Input: part model. Units: mm. Frame: model coordinates. Give positions to 0.01 mm unless a question says otherwise; leave off trailing zeros. Loops run counter-clockwise (first coordinate to the right, second up) from the corner with the lowest first, then second, coordinate; pieces in that order, holes last. Notation, with made-up numbers: M -30.75,-31 L 21.25,-31 A22 cw 21.25,-7 Z; hole C -0.5,11 d5. An arc over 180 degrees is marked long. Use CSV: the item, a comma, the result in double quotes. Start each with the question number.
Q1. Pin query (flat end, axial travel): pin 1 (1.1 mm diameter, centred on x = 0, z = 86.5, fed in from +Y); pin 2 (1.1 mm diameter, centred on y = -0.5, z = 83.5, fed in from +X); pin 3 (1.8 mm diameter, centred on x = 0, z = 88.5, fed in from -Y). Return the tip coordinate at first contact, or that it passes through.
Q2. Section A-A, the plane x = 0. Output: boundary loops of the cut face in (y, z).
Q3. Material intervals for line 1 along Y through (x, z) = (0, 107.5); line 2 along Y through (x, z) = (5.5, 63.5); line 3 along X through (y, z) = (3.25, 27), sorted ascending.
Autodesk Inventor part; units mm, degrees
ref_plane "Start Plane" through (0, 0, 10.031) normal (0, 0, 1) x (1, 0, 0)
ref_plane "End Plane" through (0, 0, 139.969) normal (0, 0, 1) x (1, 0, 0)
ref_plane "Work Plane6" through (-500, 9, 10.031) normal (0, 0, -1) x (-1, 0, 0)
ref_plane "Start Plane" through (0, 0, 10.031) normal (0, 0, 1) x (1, 0, 0)
ref_plane "End Plane" through (0, 0, 139.969) normal (0, 0, 1) x (1, 0, 0)
sketch "Sketch" plane through (0, 0, 0) normal (0, 0, 1) x (1, 0, 0)
  line L0 (0, 0) -> (2.5, 0) construction
  line L1 (0, 0) -> (0, 2.5) construction
  line L2 (0, 4) -> (0, -4) construction
  line L3 (0, 4) -> (1.7574, 4)
  arc A0 (1.7574, 4) -> (3.1716, 4.5858) centre (1.7574, 6) ccw
  line L4 (3.1716, 4.5858) -> (5.7322, 7.1464)
  line L5 (-4, 0) -> (4, 0) construction
  line L6 (4, 0) -> (4, 1.7574)
  arc A1 (4.5858, 3.1716) -> (4, 1.7574) centre (6, 1.7574) ccw
  line L7 (4.5858, 3.1716) -> (7.1464, 5.7322)
  line L8 (0, 0) -> (10, 10) construction
  line L9 (0, 0) -> (19.6827, 0) construction
  arc A2 (8, 5.3787) -> (7.1464, 5.7322) centre (7.5, 5.3787) ccw
  line L10 (8, 5.3787) -> (8, 3.5)
  arc A3 (8, 3.5) -> (8.5, 3) centre (8.5, 3.5) ccw
  line L11 (8.5, 3) -> (9.5, 3)
  arc A4 (9.5, 3) -> (10, 3.5) centre (9.5, 3.5) ccw
  line L12 (10, 3.5) -> (10, 9)
  line L13 (10, 9) -> (10, 10) construction
  arc A5 (5.7322, 7.1464) -> (5.3787, 8) centre (5.3787, 7.5) ccw
  line L14 (5.3787, 8) -> (3.5, 8)
  arc A6 (3, 8.5) -> (3.5, 8) centre (3.5, 8.5) ccw
  line L15 (3, 8.5) -> (3, 9.5)
  arc A7 (3.5, 10) -> (3, 9.5) centre (3.5, 9.5) ccw
  line L16 (3.5, 10) -> (9, 10)
  arc A8 (10, 9) -> (9, 10) centre (9, 9) ccw
  line L17 (0, 4) -> (-1.7574, 4)
  arc A9 (-3.1716, 4.5858) -> (-1.7574, 4) centre (-1.7574, 6) ccw
  line L18 (-3.1716, 4.5858) -> (-5.7322, 7.1464)
  line L19 (-4, 0) -> (-4, 1.7574)
  arc A10 (-4, 1.7574) -> (-4.5858, 3.1716) centre (-6, 1.7574) ccw
  line L20 (-4.5858, 3.1716) -> (-7.1464, 5.7322)
  arc A11 (-7.1464, 5.7322) -> (-8, 5.3787) centre (-7.5, 5.3787) ccw
  line L21 (-8, 5.3787) -> (-8, 3.5)
  arc A12 (-8.5, 3) -> (-8, 3.5) centre (-8.5, 3.5) ccw
  line L22 (-8.5, 3) -> (-9.5, 3)
  arc A13 (-10, 3.5) -> (-9.5, 3) centre (-9.5, 3.5) ccw
  line L23 (-10, 3.5) -> (-10, 9)
  arc A14 (-5.3787, 8) -> (-5.7322, 7.1464) centre (-5.3787, 7.5) ccw
  line L24 (-5.3787, 8) -> (-3.5, 8)
  arc A15 (-3.5, 8) -> (-3, 8.5) centre (-3.5, 8.5) ccw
  line L25 (-3, 8.5) -> (-3, 9.5)
  arc A16 (-3, 9.5) -> (-3.5, 10) centre (-3.5, 9.5) ccw
  line L26 (-3.5, 10) -> (-9, 10)
  arc A17 (-9, 10) -> (-10, 9) centre (-9, 9) ccw
  line L27 (0, -4) -> (-1.7574, -4)
  arc A18 (-1.7574, -4) -> (-3.1716, -4.5858) centre (-1.7574, -6) ccw
  line L28 (-3.1716, -4.5858) -> (-5.7322, -7.1464)
  arc A19 (-5.7322, -7.1464) -> (-5.3787, -8) centre (-5.3787, -7.5) ccw
  line L29 (-5.3787, -8) -> (-3.5, -8)
  arc A20 (-3, -8.5) -> (-3.5, -8) centre (-3.5, -8.5) ccw
  line L30 (-3, -8.5) -> (-3, -9.5)
  arc A21 (-3.5, -10) -> (-3, -9.5) centre (-3.5, -9.5) ccw
  line L31 (-3.5, -10) -> (-9, -10)
  arc A22 (-10, -9) -> (-9, -10) centre (-9, -9) ccw
  line L32 (-10, -3.5) -> (-10, -9)
  arc A23 (-9.5, -3) -> (-10, -3.5) centre (-9.5, -3.5) ccw
  line L33 (-8.5, -3) -> (-9.5, -3)
  arc A24 (-8, -3.5) -> (-8.5, -3) centre (-8.5, -3.5) ccw
  line L34 (-8, -5.3787) -> (-8, -3.5)
  arc A25 (-8, -5.3787) -> (-7.1464, -5.7322) centre (-7.5, -5.3787) ccw
  line L35 (-4.5858, -3.1716) -> (-7.1464, -5.7322)
  arc A26 (-4.5858, -3.1716) -> (-4, -1.7574) centre (-6, -1.7574) ccw
  line L36 (-4, 0) -> (-4, -1.7574)
  line L37 (3.5, -10) -> (9, -10)
  arc A27 (9, -10) -> (10, -9) centre (9, -9) ccw
  line L38 (10, -3.5) -> (10, -9)
  arc A28 (10, -3.5) -> (9.5, -3) centre (9.5, -3.5) ccw
  line L39 (8.5, -3) -> (9.5, -3)
  arc A29 (8.5, -3) -> (8, -3.5) centre (8.5, -3.5) ccw
  line L40 (8, -5.3787) -> (8, -3.5)
  arc A30 (7.1464, -5.7322) -> (8, -5.3787) centre (7.5, -5.3787) ccw
  line L41 (4.5858, -3.1716) -> (7.1464, -5.7322)
  arc A31 (4, -1.7574) -> (4.5858, -3.1716) centre (6, -1.7574) ccw
  line L42 (4, 0) -> (4, -1.7574)
  line L43 (5.3787, -8) -> (3.5, -8)
  arc A32 (5.3787, -8) -> (5.7322, -7.1464) centre (5.3787, -7.5) ccw
  line L44 (3.1716, -4.5858) -> (5.7322, -7.1464)
  arc A33 (3.1716, -4.5858) -> (1.7574, -4) centre (1.7574, -6) ccw
  line L45 (0, -4) -> (1.7574, -4)
  arc A34 (3.5, -8) -> (3, -8.5) centre (3.5, -8.5) ccw
  line L46 (3, -8.5) -> (3, -9.5)
  arc A35 (3, -9.5) -> (3.5, -10) centre (3.5, -9.5) ccw
  circle A36 centre (0, 0) radius 2.5
  dimension "d1" = 8
  dimension "d2" = 2
  dimension "d3" = 8
  dimension "d4" = 2
  dimension "d5" = 2
  dimension "d7" = 45
  dimension "d8" = 0.5
  dimension "d9" = 0.5
  dimension "d10" = 0.5
  dimension "d12" = 2
  dimension "d17" = 7
  dimension "d18" = 10
  dimension "d19" = 0.5
  dimension "d20" = 1
  dimension "d21" = 0.5
  dimension "d22" = 0.5
  dimension "d23" = 2
  dimension "d24" = 7
  dimension "d25" = 5
extrude "Body" add sketch "Sketch" along normal up to surface (129.938 mm away) from surface at 10.031
sketch "Sketch6" plane through (0, 0, 0) normal (0, 0, 1) x (1, 0, 0)
  line L0 (0, 0) -> (10, 0)
ref_plane "Work Plane5" through (0, 0, 0) normal (0, -1, 0) x (1, 0, 0)
sketch "Sketch7" plane through (0, 0, 0) normal (0, -1, 0) x (1, 0, 0)
  line L0 (-2, 10.031) -> (12, 10.031)
  line L1 (-2, 139.969) -> (12, 139.969)
  dimension "d33" = 129.938
ref_plane "Work Plane6" through (-500, 9, 10.031) normal (0, 0, -1) x (-1, 0, 0)
split "Split1" plane through (-500, 9, 10.031) removes the side toward (0, 0, -1)
ref_plane "Work Plane7" through (0, 9, 139.969) normal (0, 0, 1) x (1, 0, 0)
split "Split2" plane through (0, 9, 139.969) removes the side toward (0, 0, 1)
ref_plane "Work Plane8" through (-500, 0, 10.031) normal (0, 0, -1) x (-1, 0, 0)
split "Split3" plane through (-500, 0, 10.031) removes the side toward (0, 0, -1)
ref_plane "Work Plane9" through (0, 0, 139.969) normal (0, 0, 1) x (1, 0, 0)
split "Split4" plane through (0, 0, 139.969) removes the side toward (0, 0, 1)
equation "\"d1\" = 0.8 * sigma"
equation "\"d2\" = 0.2 * sigma"
equation "\"d3\" = 0.8 * sigma"
equation "\"d4\" = 0.2 * sigma"
equation "\"d5\" = 0.2 * sigma"
equation "\"d8\" = 0.05 * sigma"
equation "\"d9\" = 0.05 * sigma"
equation "\"d10\" = 0.05 * sigma"
equation "\"d12\" = 0.2 * sigma"
equation "\"d17\" = 0.7 * sigma"
equation "\"d18\" = sigma"
equation "\"d19\" = 0.05 * sigma"
equation "\"d20\" = 0.1 * sigma"
equation "\"d21\" = 0.05 * sigma"
equation "\"d22\" = 0.05 * sigma"
equation "\"d23\" = 0.2 * sigma"
equation "\"d24\" = 0.7 * sigma"
equation "\"d25\" = 0.5 * sigma"
equation "\"sigma\" = 1"
equation "\"G_OFFSET_START\" = -10.031"
equation "\"G_OFFSET_END\" = -10.031"
equation "\"d28\" = -G_OFFSET_START"
equation "\"d29\" = Length + G_OFFSET_END"
equation "\"G_L\" = d33"
properties part number "A3.3-MEM"
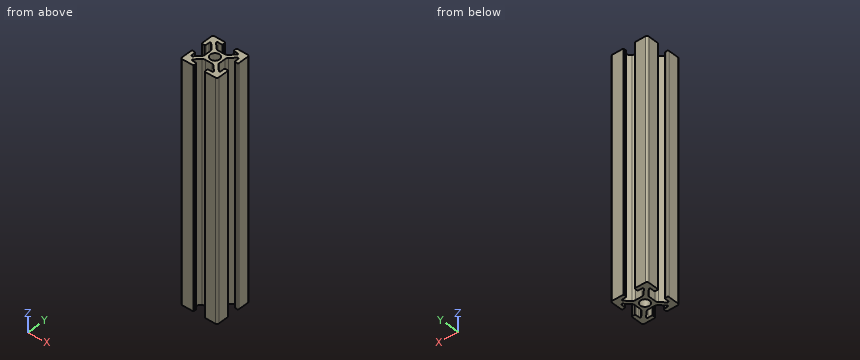
A:
1,pin 1,"y = 4"
1,pin 2,"x = 4"
1,pin 3,"y = -4"
2,outline,"M -4,10.03 L -2.5,10.03 L -2.5,139.97 L -4,139.97 Z; M 2.5,10.03 L 4,10.03 L 4,139.97 L 2.5,139.97 Z"
3,line 1,"-4 to -2.5, 2.5 to 4"
3,line 2,"-10 to -7.99, -6.91 to -4.09, 4.09 to 6.91, 7.99 to 10"
3,line 3,"-9.93 to -8.07, -4.66 to 4.66, 8.07 to 9.93"
